Part model, mm, in its own coordinate system. A direction names the side the tool comes from. Round coordinates to 2 decimals unless told otherwise and drop trailing zeros. Write each loop counter-clockwise with the first axis right and the second up, starting at its lowest first coordinate (ties: lowest second). Pieces come first, ordered by that corner, then holes. Notation, with made-up numbers: M 14.25,24 L 43.25,24 A19 cw 43.25,42 Z; hole C 11,83.25 d1. An arc over 180 degrees is marked long. Answer as a JSON object with one key per item and string values. Group by question number.
1. Drop flat-ended pins along their axis: pin 1 (2 mm diameter, centred on x = 5, z = 1, fed in from -Y); pin 2 (1 mm diameter, centred on x = 8.5, y = -13.5, fed in from +Z); pin 3 (2 mm diameter, centred on x = 1.5, z = 5, fed in from -Y). Give the stop position or say it passes through.
2. Which spindle directions (+Z, -Z, +X, -X, +Y, -Y) get a long thin tool onto all of the face, cutting with end or side? Do faces 4 (the face through (23.813, 2.083, 4.035)), 5 (the face through (-23.813, 2.083, 4.035)), 6 (the face through (-2.083, -23.813, 4.035)). Say none if no direction does.
3. Drill centre lines: line 1 (Z direction, x = 8, y = -18); line 2 (X direction, y = 10.5, z = 5.25); line 3 (Y direction, x = -10, z = 6.25). Where is each one in solid material? Low to high. Write a range as from..to.
4. Band-saw the part on A-A, the plane z = 3.5. Write the cut outline in (x, y).
5. Two-plate mould, pull along Y, no slides. Class faces 1 (the face through (17.539, 17.885, 3.423)), 2 (the face through (-17.539, -17.885, 3.423)), 3 (the face through (0, 0, 1.5)): +Y half, -Y half, draft (parallel to the pull), parting line (faces both ways), or undercut.
6. Band-saw the part on B-B, the plane x = 0. Write the cut outline in (y, z), plus the area to 3 significant figures.
from build123d import *

# Parameters (mm, degrees)
F2_SIZE2        = 1.0989909678
F2_SIZE         = 0.4
F4_R            = 1
F3_W            = 7.3154903948
F3_H            = 6.1171914935
F5_ANGLE_BACK   = 5
F5_ANGLE        = 10
F5_COPIES_COUNT = 4
F6_R            = 0.3


# Not quite as in the source:
# - a pattern or mirror of a feature is missing from the dataset's text; its kind, count and spacing are read off the source's solid


with BuildPart() as f1:
    # F0 (on Front) → F1 (revolve)
    with BuildSketch(Plane.XZ):
        Polygon((-28.3, 0), (0, 0), (0, 1.5), (-23.05, 1.5), (-23.05, 6.5), (-25.05, 6.5), (-25.05, 1.5), (-28.3, 1.5), align=None)
    revolve(axis=Axis((0, 0, -0.5399994552), (0, 0, -1)))

    # F2
    f2_edges = [f1.edges().sort_by_distance(p)[0] for p in [
        (25.05, 0, 6.5),
    ]]
    chamfer(f2_edges, length=F2_SIZE, length2=F2_SIZE2)

    # F4
    f4_edges = [f1.edges().sort_by_distance(p)[0] for p in [
        (23.05, 0, 1.5),
    ]]
    fillet(f4_edges, radius=F4_R)

    # F3 (on Front) → F5 (revolve, cut)
    with BuildSketch(Plane.XZ, mode=Mode.PRIVATE) as f5_sk:
        with Locations((-22.2290772945, 4.5585957468)):
            Rectangle(F3_W, F3_H)
    f5 = revolve(f5_sk.sketch.rotate(Axis((0, 0, 7.0531656966), (0, 0, 1)), -F5_ANGLE_BACK), axis=Axis((0, 0, 7.0531656966), (0, 0, 1)), revolution_arc=F5_ANGLE, mode=Mode.SUBTRACT)

    # F5_copies: F5 ×4 about axis
    f5_copies_axis = Axis((0, 0, 0), (0, 0, 1))
    for i in range(1, F5_COPIES_COUNT):
        add(f5.rotate(f5_copies_axis, i * 360 / F5_COPIES_COUNT), mode=Mode.SUBTRACT)

    # F6
    f6_edges = [f1.edges().sort_by_distance(p)[0] for p in [
        (28.3, 0, 1.5),
        (28.3, 0, 0),
    ]]
    fillet(f6_edges, radius=F6_R)


solid = f1.part
Worked answers:
{
 "1": {"pin 1": "stops at y = -28.02", "pin 2": "stops at z = 1.5", "pin 3": "stops at y = -24.95"},
 "2": {"face 4": "+Z, +X", "face 5": "+Z, -X", "face 6": "+Z, -Y"},
 "3": {"line 1": "z = 0..1.5", "line 2": "x = -22.74..-20.52, 20.52..22.74", "line 3": "y = -22.63..-20.77, 20.77..22.63"},
 "4": {"outline": "M -24.95,-2.18 A25.05 ccw -2.18,-24.95 L -2.01,-22.96 A23.05 cw -22.96,-2.01 Z; M -24.95,2.18 L -22.96,2.01 A23.05 cw -2.01,22.96 L -2.18,24.95 A25.05 ccw Z; M 2.01,-22.96 L 2.18,-24.95 A25.05 ccw 24.95,-2.18 L 22.96,-2.01 A23.05 cw Z; M 2.01,22.96 A23.05 cw 22.96,2.01 L 24.95,2.18 A25.05 ccw 2.18,24.95 Z"},
 "5": {"face 1": "+Y half", "face 2": "-Y half", "face 3": "undercut"},
 "6": {"outline": "M -28.3,0.3 A0.3 ccw -28,0 L 28,0 A0.3 ccw 28.3,0.3 L 28.3,1.2 A0.3 ccw 28,1.5 L -28,1.5 A0.3 ccw -28.3,1.2 Z", "area": "84.8 mm^2"}
}
